Here's how the part is built. I have some questions about the finished solid (model axes, mm). A direction names the side the tool comes from. Coordinates: 2 decimals unless noted, no trailing zeros. Order: outer loops, then holes, each group sorted by start corner. A loop starts at its lowest first (then second) coordinate and runs counter-clockwise, first axis right, second up. Notation, with made-up numbers: (-29.75, 10) - (18.25, 10) arc R8 ccw to (18.25, 14) - close; hole circle Ø10 at (71.25, 74). An arc over 180 degrees is marked (long way). Use CSV: the item, a comma, the result in double quotes. Start each with the question number.
from build123d import *

# Parameters (mm, degrees)
F0_R     = 3.3
F0_R_2   = 10
F1_DEPTH = 26
F2_SIZE  = 1
F3_SIZE  = 2
F4_R     = 7
F4_R_2   = 4.5
F5_DEPTH = 8.5
F6_DEPTH = 50.001


with BuildPart() as f1:
    # F0 (on Front) → F1 (new body)
    with BuildSketch(Plane.XZ):
        Polygon((-26.441849, 23.418281), (-44.441849, 23.418281), (-44.441849, -26.581719), (43.558151, -26.581719), (43.558151, 23.418281), (25.558151, 23.418281), (25.558151, 33.418281), (-26.441849, 33.418281), align=None)
        with Locations((-33.048104, -14.581719)):
            Circle(F0_R, mode=Mode.SUBTRACT)
        with Locations((34.650207, -14.581719)):
            Circle(F0_R, mode=Mode.SUBTRACT)
        with Locations((-34.040019, 7.418281)):
            Circle(F0_R, mode=Mode.SUBTRACT)
        with Locations((-0.441849, 7.418281)):
            Circle(F0_R_2, mode=Mode.SUBTRACT)
        with Locations((35.394143, 7.418281)):
            Circle(F0_R, mode=Mode.SUBTRACT)
    extrude(amount=F1_DEPTH)

    # F2
    f2_edges = [f1.edges().sort_by_distance(p)[0] for p in [
        (-44.441849, -13, 23.418281),
        (43.558151, -13, 23.418281),
    ]]
    chamfer(f2_edges, length=F2_SIZE)

    # F3
    f3_edges = [f1.edges().sort_by_distance(p)[0] for p in [
        (-26.441849, -13, 33.418281),
        (25.558151, -13, 33.418281),
    ]]
    chamfer(f3_edges, length=F3_SIZE)

    # F4 (on face) → F5 (cut)
    with BuildSketch(Plane.XY.offset(23.418281)):
        with Locations((-35.441849, -13.069903)):
            Circle(F4_R)
        with Locations((-35.441849, -13.069903)):
            Circle(F4_R_2, mode=Mode.SUBTRACT)
        with Locations((34.558151, -12.861175)):
            Circle(F4_R)
        with Locations((34.558151, -12.861175)):
            Circle(F4_R_2, mode=Mode.SUBTRACT)
    extrude(amount=-F5_DEPTH, mode=Mode.SUBTRACT)

    # F4 (on face) → F6 (cut, through all)
    with BuildSketch(Plane.XY.offset(23.418281)):
        with Locations((-35.441849, -13.069903)):
            Circle(F4_R_2)
        with Locations((34.558151, -12.861175)):
            Circle(F4_R_2)
    extrude(amount=-F6_DEPTH, mode=Mode.SUBTRACT)


solid = f1.part
Item 1: For pin 1 Ø8 at (y, z) = (-7, 25.5) entering from -X; pin 2 Ø6.5 at (y, z) = (-19, 28.5) entering from -X; pin 3 Ø6 at (x, z) = (34.65, -14.58) entering from -Y; pin 4 Ø11.5 at (x, y) = (-35.44, -13.07) entering from +Z, each with a flat end and sliding along its axis, tell me the tip position at first contact or that it passes through.
Item 2: Suppose I cut it at A-A on z = 12.5. Write out the boundary of the cut face in (x, y).
Item 3: For faces 1 (the flat face through (43.558, -13, -2)), 2 (the flat face through (30, -19, 23.418)), 3 (the cylindrical face through (-42.435, -12.762, 19.228)), 4 (the flat face through (-31, -7, 23.418)), which set-ups out of +Z, -Z, +X, -X, +Y, -Y let a thin tool reach every point of the face, with its end or its side?
Item 4: Suppose I cut it at C-C on y = -24. Write out the boundary of the cut face in (x, z).
Item 5: Suppose I cut it at B-B on x = 7. Write out the boundary of the cut face in (y, z), then the cut area to 3 significant figures.
Item 6: Please list where these lines run through material, in increasing order: line 1 along X through (y, z) = (-13, -19); line 2 along X through (y, z) = (-19.5, 10); line 3 along X through (y, z) = (-17, 2). Write a range as from..to.
Item 7: We'd pull the mould along Y, two halves only. Please class faces 5 (the flat face through (-1, 0, -3)), 6 (the flat face through (-36, -18, 14.918)), 7 (the cylindrical face through (-29.9, -12.82, -13.59)): released by +Y, released by -Y, zero draft, split by the parting line, or undercut.
Item 8: Suppose I cut it at D-D on z = -13.5. Write out the boundary of the cut face in (x, y).
Here are the results:
1,pin 1,"x = -44.44"
1,pin 2,"x = -26.44"
1,pin 3,"through"
1,pin 4,"z = 14.92"
2,outline,"(-44.44, -26) - (-9.05, -26) - (-9.05, 0) - (-44.44, 0) - close; (8.17, -26) - (43.56, -26) - (43.56, 0) - (8.17, 0) - close; hole circle Ø9 at (-35.44, -13.07); hole circle Ø9 at (34.56, -12.86)"
3,face 1,"+Z, -Z, +X, +Y, -Y"
3,face 2,"+Z, +X, +Y, -Y"
3,face 3,"+Z"
3,face 4,"+Z, -X, +Y, -Y"
4,outline,"(-44.44, -26.58) - (43.56, -26.58) - (43.56, 22.42) - (42.56, 23.42) - (25.56, 23.42) - (25.56, 31.42) - (23.56, 33.42) - (-24.44, 33.42) - (-26.44, 31.42) - (-26.44, 23.42) - (-43.44, 23.42) - (-44.44, 22.42) - close; hole circle Ø6.6 at (-34.04, 7.42); hole circle Ø6.6 at (-33.05, -14.58); hole circle Ø20 at (-0.44, 7.42); hole circle Ø6.6 at (34.65, -14.58); hole circle Ø6.6 at (35.39, 7.42)"
5,outline,"(-26, -26.58) - (0, -26.58) - (0, 0.74) - (-26, 0.74) - close; (-26, 14.1) - (0, 14.1) - (0, 33.42) - (-26, 33.42) - close"
5,area,"1,210 mm^2"
6,line 1,"-44.44..-39.94, -30.94..30.06, 39.06..43.56"
6,line 2,"-44.44..-36.1, -31.98..-10.1, 9.22..33.34, 37.45..43.56"
6,line 3,"-44.44..-37.63, -33.25..-8.85, 7.96..32.79, 36.32..43.56"
7,face 5,"released by +Y"
7,face 6,"undercut"
7,face 7,"zero draft"
8,outline,"(-44.44, -26) - (-36.17, -26) - (-36.17, -17.51) arc R4.5 cw to (-36.17, -8.63) - (-36.17, 0) - (-44.44, 0) - close; (-29.93, -26) - (31.53, -26) - (31.53, -16.19) arc R4.5 cw to (31.53, -9.53) - (31.53, 0) - (-29.93, 0) - close; (37.77, -26) - (43.56, -26) - (43.56, 0) - (37.77, 0) - (37.77, -9.71) arc R4.5 cw to (37.77, -16.02) - close"
